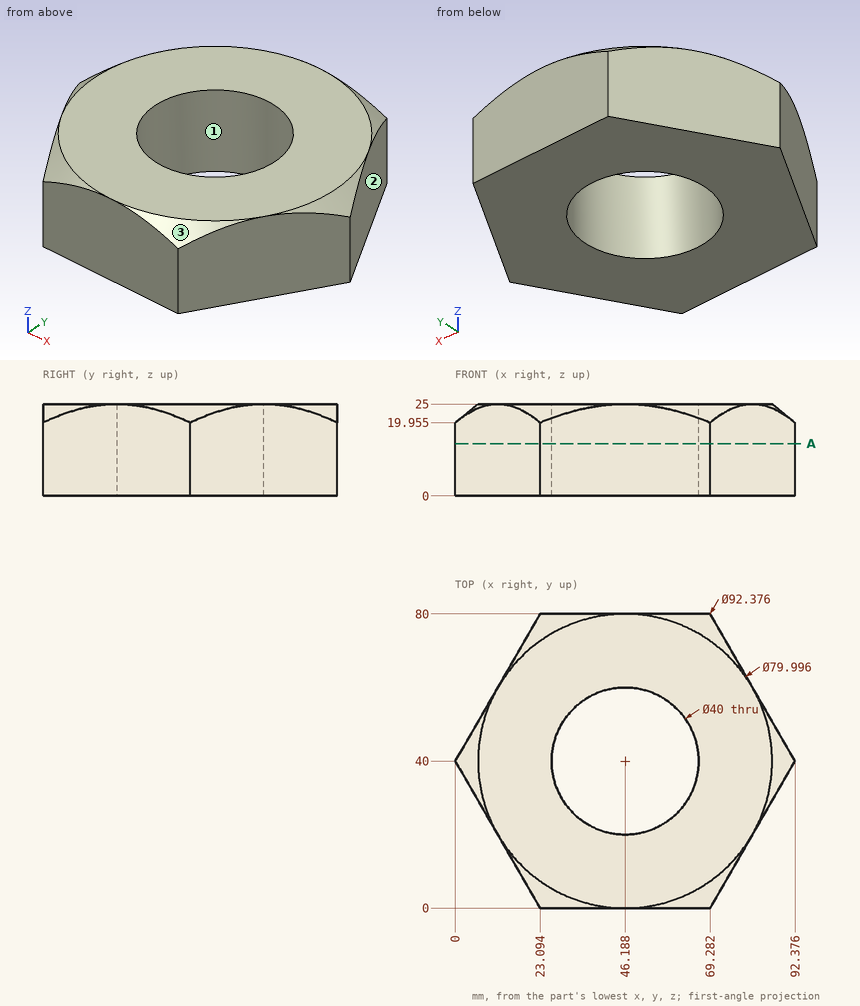
For this review, use the dimensioned drawing (mm, ordinates from the lowest corner) and the shaded views. Give positions to 0.01 mm unless a question says otherwise; leave off trailing zeros. Order: outer loops, then holes, each group sorted by start corner. A loop starts at its lowest first (then second) coordinate and runs counter-clockwise, first axis right, second up. Notation, with made-up numbers: M 33,59.5 L 70,59.5 A24 cw 70,98.5 Z; hole C 57,85.25 d2. An arc over 180 degrees is marked long. One line per question, with ' | ' between items. Start each with the question number.
1) Consider section A-A, the plane z = 14.25. Give the boundary of the cut face in (x, y).
2) Wall thickness on L1, parallel to X at y = 32, z = 1.25; L2, parallel to Y at x = 61.5, z = 5.75; L3, parallel to Y at x = 37, z = 20.25: over which ranges is each line inside the solid? List them lowest first. Write a range as from..to.
3) Mouldability with a two-part tool opening along X and no side actions: class the marked faces 1, 2 and 3 as pulls with the +X half, pulls with the -X half, needs draft (parallel to the pull), parting line crosses it, or undercut.
4) Clearance check with flat-ended pins moving along their axes: P1, Ø1, axis at x = 73, z = 9.5, coming from the +Y side; P2, Ø12, axis at y = 11.5, z = 14.5, coming from the +X side; P3, Ø5, axis at y = 33, z = 19.5, coming from the -X side. State where each tip first meets the part, or that it passes through.
Found:
1) outline: M 0,40 L 23.09,0 L 69.28,0 L 92.38,40 L 69.28,80 L 23.09,80 Z; hole C 46.19,40 d40
2) L1: x = 4.62..27.86, 64.52..87.76 | L2: y = 0..27.13, 52.87..80 | L3: y = 0..22.24, 57.76..80
3) face 1: undercut | face 2: pulls with the +X half | face 3: parting line crosses it
4) P1: stops at y = 74.43 | P2: stops at x = 79.39 | P3: stops at x = 2.6
